Verification items for the finished model (mm, model axes). Face numbers are marked on the shaded views. A direction names the side the tool comes from. Give positions to 0.01 mm unless a question says otherwise; leave off trailing zeros. Write each loop counter-clockwise with the first axis right and the second up, starting at its lowest first coordinate (ties: lowest second). Pieces come first, ordered by that corner, then holes. Notation, with made-up numbers: (13, -37) -> (55, -37) arc R4 ccw to (55, -33) -> close; hole circle Ø6 at (79, -9.5). An arc over 180 degrees is marked (long way). Answer as CSV lines item,"result". Start each with the question number.
1) Tool access check on the marked faces 1 and 2. Record the directions out of +Z, -Z, +X, -X, +Y, -Y that give a thin tool (end or side, any length) a straight path to the whole face; none if there is none.
2) Sectioned sample at D-D on x = -15.5. Record the cut outline in (y, z).
3) Material ranges on L1, parallel to X at y = 13.9, z = 0; L2, parallel to X at y = 7, z = 0; L3, parallel to X at y = 3, z = -15.5, recorded low to high.
4) Sectioned sample at C-C on y = 7.75. Give the number of separate pieces and of enclosed holes in the cut face, and give its area (3 significant figures).
5) Gauge pin test, flat ends, axial feed: pin 1 Ø1.5 at (y, z) = (2.5, 10.5) entering from +X; pin 2 Ø1.5 at (x, y) = (2.5, 13) entering from -Z; pin 3 Ø2 at (x, z) = (15.5, -1.5) entering from +Y; pin 4 Ø4 at (x, z) = (15, -5) entering from -Y. Record the tip position at first contact, or that the pin passes through.
6) Sectioned sample at B-B on z = 0. Record the cut outline in (x, y).
7) Mould release check, pull along Z, two halves, no side actions. Record for the marked faces 3, 4, 5 and 6: released by +Z, released by -Z, zero draft, split by the parting line, or undercut.
8) Sectioned sample at A-A on x = 0. Record the cut outline in (y, z).
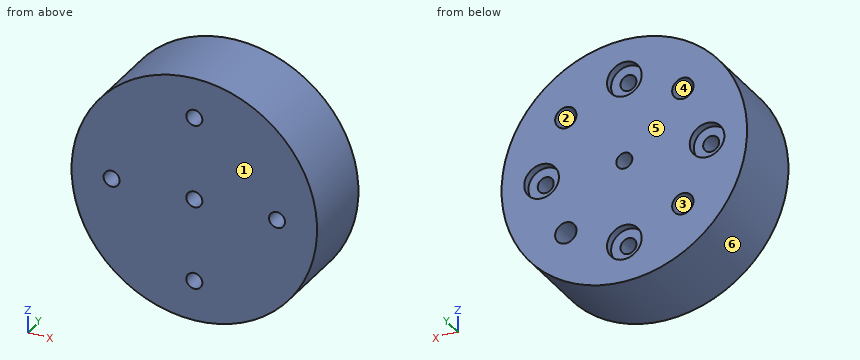
```python
from build123d import *

# Parameters (mm, degrees)
SKETCH1_R           = 23
SKETCH1_R_2         = 1.5
BOSS_EXTRUDE1_DEPTH = 15
SKETCH2_R           = 3.25
CUT_EXTRUDE1_DEPTH  = 1.5
SKETCH3_R           = 2
CUT_EXTRUDE2_DEPTH  = 10


with BuildPart() as part:
    # Sketch1 → Boss-Extrude1 (new body)
    with BuildSketch(Plane(origin=(0, 0, 0), x_dir=(1, 0, 0), z_dir=(0, 1, 0))):
        with Locations(Location((0, 0, 0), (0, 0, 270))):
            Circle(SKETCH1_R)
        with Locations(Location((0, 15.5, 0), (0, 0, 270))):
            Circle(SKETCH1_R_2, mode=Mode.SUBTRACT)
        with Locations(Location((15.5, 0, 0), (0, 0, 270))):
            Circle(SKETCH1_R_2, mode=Mode.SUBTRACT)
        with Locations(Location((0, -15.5, 0), (0, 0, 270))):
            Circle(SKETCH1_R_2, mode=Mode.SUBTRACT)
        with Locations(Location((-15.5, 0, 0), (0, 0, 270))):
            Circle(SKETCH1_R_2, mode=Mode.SUBTRACT)
        with Locations(Location((0, 0, 0), (0, 0, 270))):
            Circle(SKETCH1_R_2, mode=Mode.SUBTRACT)
    extrude(amount=BOSS_EXTRUDE1_DEPTH)

    # Sketch2 → Cut-Extrude1 (cut)
    with BuildSketch(Plane(origin=(0, 15, 0), x_dir=(1, 0, 0), z_dir=(0, 1, 0))):
        with Locations(Location((0, 15.5, 0), (0, 0, 270))):
            Circle(SKETCH2_R)
        with Locations(Location((15.5, 0, 0), (0, 0, 270))):
            Circle(SKETCH2_R)
        with Locations(Location((0, -15.5, 0), (0, 0, 270))):
            Circle(SKETCH2_R)
        with Locations(Location((-15.5, 0, 0), (0, 0, 270))):
            Circle(SKETCH2_R)
    extrude(amount=-CUT_EXTRUDE1_DEPTH, mode=Mode.SUBTRACT)

    # Sketch3 → Cut-Extrude2 (cut)
    with BuildSketch(Plane(origin=(0, 15, 0), x_dir=(1, 0, 0), z_dir=(0, 1, 0))):
        with Locations(Location((-10.960155108, 10.960155108, 0), (0, 0, 270))):
            Circle(SKETCH3_R)
        with Locations(Location((10.960155108, 10.960155108, 0), (0, 0, 270))):
            Circle(SKETCH3_R)
        with Locations(Location((10.960155108, -10.960155108, 0), (0, 0, 270))):
            Circle(SKETCH3_R)
        with Locations(Location((-10.960155108, -10.960155108, 0), (0, 0, 270))):
            Circle(SKETCH3_R)
    extrude(amount=-CUT_EXTRUDE2_DEPTH, mode=Mode.SUBTRACT)


solid = part.part
```
Ans:
1,face 1,"+Z, -Z, +X, -X, -Y"
1,face 2,"+Y"
2,outline,"(0, -16.99) -> (15, -16.99) -> (15, -3.25) -> (13.5, -3.25) -> (13.5, -1.5) -> (0, -1.5) -> close; (0, 1.5) -> (13.5, 1.5) -> (13.5, 3.25) -> (15, 3.25) -> (15, 16.99) -> (0, 16.99) -> close"
3,L1,"x = -23 to -18.75, -12.25 to -1.5, 1.5 to 12.25, 18.75 to 23"
3,L2,"x = -23 to -17, -14 to -1.5, 1.5 to 14, 17 to 23"
3,L3,"x = -16.99 to -1.5, 1.5 to 16.99"
4,separate pieces,"1"
4,enclosed holes,"9"
4,area,"1,580 mm²"
5,pin 1,"stops at x = 20.83"
5,pin 2,"stops at z = -22.93"
5,pin 3,"stops at y = 13.5"
5,pin 4,"stops at y = 0"
6,outline,"(-23, 0) -> (-17, 0) -> (-17, 13.5) -> (-18.75, 13.5) -> (-18.75, 15) -> (-23, 15) -> close; (-14, 0) -> (-1.5, 0) -> (-1.5, 15) -> (-12.25, 15) -> (-12.25, 13.5) -> (-14, 13.5) -> close; (1.5, 0) -> (14, 0) -> (14, 13.5) -> (12.25, 13.5) -> (12.25, 15) -> (1.5, 15) -> close; (17, 0) -> (23, 0) -> (23, 15) -> (18.75, 15) -> (18.75, 13.5) -> (17, 13.5) -> close"
7,face 3,"undercut"
7,face 4,"undercut"
7,face 5,"zero draft"
7,face 6,"split by the parting line"
8,outline,"(0, -23) -> (15, -23) -> (15, -18.75) -> (13.5, -18.75) -> (13.5, -17) -> (0, -17) -> close; (0, -14) -> (13.5, -14) -> (13.5, -12.25) -> (15, -12.25) -> (15, -1.5) -> (0, -1.5) -> close; (0, 1.5) -> (15, 1.5) -> (15, 12.25) -> (13.5, 12.25) -> (13.5, 14) -> (0, 14) -> close; (0, 17) -> (13.5, 17) -> (13.5, 18.75) -> (15, 18.75) -> (15, 23) -> (0, 23) -> close"
